Here's how the part is built. I have some questions about the finished solid (model axes, mm). A direction names the side the tool comes from. Round coordinates to 2 decimals unless told otherwise and drop trailing zeros. Order: outer loops, then holes, each group sorted by start corner. A loop starts at its lowest first (then second) coordinate and runs counter-clockwise, first axis right, second up.
Autodesk Fusion 360 part; units mm, degrees
sketch "Eskiz1" plane through (0, 0, 0) normal (0, 1, 0) x (1, 0, 0)
  circle A0 centre (15, -20) radius 4.5
  line L0 (0, 0) -> (30, 0)
  line L1 (30, 0) -> (30, -40)
  line L2 (30, -40) -> (0, -40)
  line L3 (0, -40) -> (0, 0)
  line L4 (30, 0) -> (40, 0)
  line L5 (40, 0) -> (40, -40)
  line L6 (40, -40) -> (30, -40)
  line L7 (30, -40) -> (30, 0)
  dimension "d3" = 9
  dimension "d13" = 40
  dimension "d25" = 10
  dimension "d31" = 30
extrude "Ekstrüde Et9" add sketch "Eskiz1" along normal blind 10 contours A0 | L0 L1 L2 L3 L7
extrude "Ekstrüde Et10" add sketch "Eskiz1" along normal blind 40 contours L1 L4 L5 L6 L7
sketch "Eskiz4" plane through (30, 0, 0) normal (-1, 0, 0) x (0, 0, 1)
  line L0 (0, 10) -> (40, 10)
  line L1 (40, 10) -> (40, 40)
  line L2 (40, 40) -> (0, 40)
  line L3 (0, 40) -> (0, 10)
  circle A0 centre (20, 25) radius 4.5
  dimension "d36" = 9
  dimension "d37" = 15
hole "Delik1" at (15.0452, 0, 20.1858) direction (0, 1, 0) diameter 7.779 depth 18 tip angle 118
hole "Delik2" at (30, 25, 20) direction (1, 0, 0) diameter 7.779 depth 18 tip angle 118
1) For faces 1 (the cylindrical face through (18.5, 5.1, 18.4)), 2 (the flat face through (15, 10, 15)), which set-ups out of +Z, -Z, +X, -X, +Y, -Y let a thin tool reach every point of the face, with its end or its side?
2) If we section it at D-D (z = 25): Write out the boundary of the cut face in (x, y).
3) If we section it at C-C (x = 27): Write out the boundary of the cut face in (y, z), plus the area to 3 significant figures.
4) We'd pull the mould along Z, two halves only. Please class faces 3 (the flat face through (29, 6, 0)), 4 (the cylindrical face through (35.07, 22.371, 17.133)), 5 (the flat face through (0, 5, 20)): +Z half, -Z half, draft (parallel to the pull), parting line (faces both ways), or undercut.
5) I'm going to push flat-ended pins straight in: pin 1 (6 mm diameter, centred on x = 15.05, z = 20.19, fed in from -Y); pin 2 (15 mm diameter, centred on y = 21, z = 23.5, fed in from -X); pin 3 (6 mm diameter, centred on x = 18, z = 30.5, fed in from +Y). Where does each tip first touch, or does it pass through?
6) If we section it at A-A (y = 25): Write out the boundary of the cut face in (x, z), plus the area to 3 significant figures.
7) I need wall thicknesses on line 1 (Z direction, x = 35, y = 25); line 2 (Y direction, x = 37.25, z = 20); line 3 (Y direction, x = 3, z = 2.5). Which ranges of each line are inside material? Lowest first, please.
8) If we section it at B-B (z = 20): Write out the boundary of the cut face in (x, y).
Solutions:
1. face 1: +Y, -Y
1. face 2: +Z, -Z, -X, +Y
2. outline: (0, 0) - (40, 0) - (40, 40) - (30, 40) - (30, 10) - (0, 10) - close
3. outline: (0, 0) - (10, 0) - (10, 40) - (0, 40) - close
3. area: 400 mm2
4. face 3: -Z half
4. face 4: undercut
4. face 5: draft
5. pin 1: passes through
5. pin 2: stops at x = 30
5. pin 3: stops at y = 10
6. outline: (30, 0) - (40, 0) - (40, 16.11) - (30, 16.11) - close; (30, 23.89) - (40, 23.89) - (40, 40) - (30, 40) - close
6. area: 322 mm2
7. line 1: z = 0 to 16.11, 23.89 to 40
7. line 2: y = 0 to 21.11, 28.89 to 40
7. line 3: y = 0 to 10
8. outline: (0, 0) - (11.16, 0) - (11.16, 10) - (0, 10) - close; (18.93, 0) - (40, 0) - (40, 21.11) - (30, 21.11) - (30, 10) - (18.93, 10) - close; (30, 28.89) - (40, 28.89) - (40, 40) - (30, 40) - close
